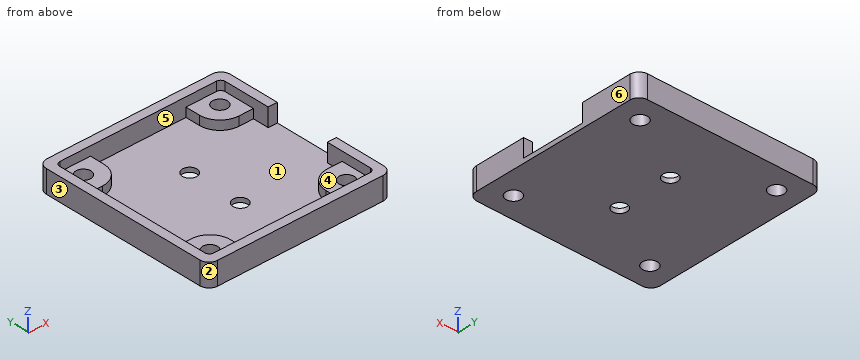
```python
from build123d import *

# Parameters (mm, degrees)
F0_R     = 1.6
F0_R_2   = 1.65
F0_W     = 2
F0_H     = 7
F1_DEPTH = 1
F2_DEPTH = 5
F3_DEPTH = 3
F4_R     = 2
F5_R     = 1


with BuildPart() as f1:
    # F0 (on Top) → F1 (new body)
    with BuildSketch(Plane.XY):
        with BuildLine():
            Line((-17.411994, -1.24302), (-17.411994, -4.438214))
            Line((-17.411994, -4.438214), (3.597618, -4.438214))
            Line((3.597618, -4.438214), (3.597618, -1.24302))
            ThreePointArc((3.597618, -1.24302), (4.915637, 1.93896), (8.097618, 3.25698))
            Line((8.097618, 3.25698), (11.292812, 3.25698))
            Line((11.292812, 3.25698), (11.292812, 6.761786))
            Line((11.292812, 6.761786), (11.292812, 13.761786))
            Line((11.292812, 13.761786), (11.292812, 20.761786))
            Line((11.292812, 20.761786), (11.292812, 24.266591))
            Line((11.292812, 24.266591), (8.097618, 24.266591))
            ThreePointArc((8.097618, 24.266591), (4.915637, 25.584611), (3.597618, 28.766591))
            Line((3.597618, 28.766591), (3.597618, 31.961786))
            Line((3.597618, 31.961786), (-17.411994, 31.961786))
            Line((-17.411994, 31.961786), (-17.411994, 28.766591))
            ThreePointArc((-17.411994, 28.766591), (-18.730013, 25.584611), (-21.911994, 24.266591))
            Line((-21.911994, 24.266591), (-25.107188, 24.266591))
            Line((-25.107188, 24.266591), (-25.107188, 3.25698))
            Line((-25.107188, 3.25698), (-21.911994, 3.25698))
            ThreePointArc((-21.911994, 3.25698), (-18.730013, 1.93896), (-17.411994, -1.24302))
        make_face()
        with Locations((-6.907188, 7.761786)):
            Circle(F0_R, mode=Mode.SUBTRACT)
        with Locations((-6.907188, 19.761786)):
            Circle(F0_R, mode=Mode.SUBTRACT)
        Polygon((-17.411994, -4.438214), (-25.107188, -4.438214), (-25.107188, 3.25698), (-25.107188, 24.266591), (-25.107188, 31.961786), (-17.411994, 31.961786), (3.597618, 31.961786), (11.292812, 31.961786), (11.292812, 24.266591), (11.292812, 20.761786), (13.292812, 20.761786), (13.292812, 33.961786), (-27.107188, 33.961786), (-27.107188, -6.438214), (13.292812, -6.438214), (13.292812, 6.761786), (11.292812, 6.761786), (11.292812, 3.25698), (11.292812, -4.438214), (3.597618, -4.438214), align=None)
        with BuildLine():
            Line((-25.107188, 31.961786), (-25.107188, 24.266591))
            Line((-25.107188, 24.266591), (-21.911994, 24.266591))
            ThreePointArc((-21.911994, 24.266591), (-18.730013, 25.584611), (-17.411994, 28.766591))
            Line((-17.411994, 28.766591), (-17.411994, 31.961786))
            Line((-17.411994, 31.961786), (-25.107188, 31.961786))
        make_face()
        with Locations((-21.911994, 28.766591)):
            Circle(F0_R_2, mode=Mode.SUBTRACT)
        with BuildLine():
            Line((11.292812, 31.961786), (3.597618, 31.961786))
            Line((3.597618, 31.961786), (3.597618, 28.766591))
            ThreePointArc((3.597618, 28.766591), (4.915637, 25.584611), (8.097618, 24.266591))
            Line((8.097618, 24.266591), (11.292812, 24.266591))
            Line((11.292812, 24.266591), (11.292812, 31.961786))
        make_face()
        with Locations((8.097618, 28.766591)):
            Circle(F0_R_2, mode=Mode.SUBTRACT)
        with Locations((12.292812, 17.261786)):
            Rectangle(F0_W, F0_H)
        with Locations((12.292812, 10.261786)):
            Rectangle(F0_W, F0_H)
    extrude(amount=F1_DEPTH)

    # F0 (on Top) → F2 (join)
    with BuildSketch(Plane.XY):
        Polygon((-17.411994, -4.438214), (-25.107188, -4.438214), (-25.107188, 3.25698), (-25.107188, 24.266591), (-25.107188, 31.961786), (-17.411994, 31.961786), (3.597618, 31.961786), (11.292812, 31.961786), (11.292812, 24.266591), (11.292812, 20.761786), (13.292812, 20.761786), (13.292812, 33.961786), (-27.107188, 33.961786), (-27.107188, -6.438214), (13.292812, -6.438214), (13.292812, 6.761786), (11.292812, 6.761786), (11.292812, 3.25698), (11.292812, -4.438214), (3.597618, -4.438214), align=None)
    extrude(amount=F2_DEPTH)

    # F0 (on Top) → F3 (join)
    with BuildSketch(Plane.XY):
        with BuildLine():
            Line((-25.107188, 31.961786), (-25.107188, 24.266591))
            Line((-25.107188, 24.266591), (-21.911994, 24.266591))
            ThreePointArc((-21.911994, 24.266591), (-18.730013, 25.584611), (-17.411994, 28.766591))
            Line((-17.411994, 28.766591), (-17.411994, 31.961786))
            Line((-17.411994, 31.961786), (-25.107188, 31.961786))
        make_face()
        with Locations((-21.911994, 28.766591)):
            Circle(F0_R_2, mode=Mode.SUBTRACT)
        with BuildLine():
            Line((-25.107188, 3.25698), (-25.107188, -4.438214))
            Line((-25.107188, -4.438214), (-17.411994, -4.438214))
            Line((-17.411994, -4.438214), (-17.411994, -1.24302))
            ThreePointArc((-17.411994, -1.24302), (-18.730013, 1.93896), (-21.911994, 3.25698))
            Line((-21.911994, 3.25698), (-25.107188, 3.25698))
        make_face()
        with Locations((-21.911994, -1.24302)):
            Circle(F0_R_2, mode=Mode.SUBTRACT)
        with BuildLine():
            Line((11.292812, 31.961786), (3.597618, 31.961786))
            Line((3.597618, 31.961786), (3.597618, 28.766591))
            ThreePointArc((3.597618, 28.766591), (4.915637, 25.584611), (8.097618, 24.266591))
            Line((8.097618, 24.266591), (11.292812, 24.266591))
            Line((11.292812, 24.266591), (11.292812, 31.961786))
        make_face()
        with Locations((8.097618, 28.766591)):
            Circle(F0_R_2, mode=Mode.SUBTRACT)
        with BuildLine():
            Line((3.597618, -1.24302), (3.597618, -4.438214))
            Line((3.597618, -4.438214), (11.292812, -4.438214))
            Line((11.292812, -4.438214), (11.292812, 3.25698))
            Line((11.292812, 3.25698), (8.097618, 3.25698))
            ThreePointArc((8.097618, 3.25698), (4.915637, 1.93896), (3.597618, -1.24302))
        make_face()
        with Locations((8.097618, -1.24302)):
            Circle(F0_R_2, mode=Mode.SUBTRACT)
    extrude(amount=F3_DEPTH)

    # F4
    f4_edges = [f1.edges().sort_by_distance(p)[0] for p in [
        (-27.107188, -6.438214, 2.5),
        (13.292812, -6.438214, 2.5),
        (13.292812, 33.961786, 2.5),
        (-27.107188, 33.961786, 2.5),
    ]]
    fillet(f4_edges, radius=F4_R)

    # F5
    f5_edges = [f1.edges().sort_by_distance(p)[0] for p in [
        (-25.107188, 31.961786, 4),
        (11.292812, 31.961786, 4),
        (11.292812, -4.438214, 4),
        (-25.107188, -4.438214, 4),
    ]]
    fillet(f5_edges, radius=F5_R)


solid = f1.part
```
Verification items for the finished model (mm, model axes). Face numbers are marked on the shaded views. A direction names the side the tool comes from. Coordinates: 2 decimals unless noted, no trailing zeros. Loops run counter-clockwise (first coordinate to the right, second up) from the corner with the lowest first, then second, coordinate; pieces in that order, holes last. Notation, with made-up numbers: (-25.5, 75) -> (-21.5, 75) arc R14 cw to (-21.5, 84) -> close; hole circle Ø11 at (62, 49.5). An arc over 180 degrees is marked (long way). Answer in a Markdown table with one row per item.
1) Draft check along Y on the marked faces 1, 2, 3 and 4. Enter one of: released by +Y, released by -Y, zero draft, split by the parting line, or undercut.
The answers:
| item | result |
|---|---|
| face 1 | undercut |
| face 2 | released by -Y |
| face 3 | zero draft |
| face 4 | undercut |
2) Access from +Z, -Z, +X, -X, +Y, -Y to the whole of each face (thin tool, end or side, straight path). Record for the marked faces 5 and 6.
The answers:
| item | result |
|---|---|
| face 5 | +Z |
| face 6 | +Z, -Z, +X, +Y, -Y |
3) Section check C-C (z = 4.1). Record the cut outline in (x, y), and give its area (3 significant figures).
The answers:
| item | result |
|---|---|
| outline | (-27.11, -4.44) arc R2 ccw to (-25.11, -6.44) -> (11.29, -6.44) arc R2 ccw to (13.29, -4.44) -> (13.29, 6.76) -> (11.29, 6.76) -> (11.29, -3.44) arc R1 cw to (10.29, -4.44) -> (-24.11, -4.44) arc R1 cw to (-25.11, -3.44) -> (-25.11, 30.96) arc R1 cw to (-24.11, 31.96) -> (10.29, 31.96) arc R1 cw to (11.29, 30.96) -> (11.29, 20.76) -> (13.29, 20.76) -> (13.29, 31.96) arc R2 ccw to (11.29, 33.96) -> (-25.11, 33.96) arc R2 ccw to (-27.11, 31.96) -> close |
| area | 277 mm2 |
4) Scan lines: line 1 along Y through (x, z) = (10, 2.5); line 2 along X through (y, z) = (29, 3.9); line 3 along Y through (x, z) = (-17, 2.7). Record each from-to range of solid material in increasing order. Write a range as from..to.
The answers:
| item | result |
|---|---|
| line 1 | y = -6.44..3.26, 24.27..33.96 |
| line 2 | x = -27.11..-25.11, 11.29..13.29 |
| line 3 | y = -6.44..-4.44, 31.96..33.96 |
5) Section check B-B (x = -10). Record the cut outline in (y, z).
The answers:
| item | result |
|---|---|
| outline | (-6.44, 0) -> (33.96, 0) -> (33.96, 5) -> (31.96, 5) -> (31.96, 1) -> (-4.44, 1) -> (-4.44, 5) -> (-6.44, 5) -> close |
6) Section check A-A (z = 1.9). Give the number of separate pieces and of enclosed holes in the cut face, and give its area (3 significant figures).
The answers:
| item | result |
|---|---|
| separate pieces | 1 |
| enclosed holes | 4 |
| area | 461 mm2 |
7) Depth check by flat-ended pin: P1, Ø1, axis at y = 10.5, z = 3, coming from the +X side; P2, Ø3, axis at x = -21.91, y = -1.24, coming from the +Z side. Enter the tip coordinate at first touch or a pass-through.
The answers:
| item | result |
|---|---|
| P1 | stops at x = -25.11 |
| P2 | passes through |
8) Section check D-D (y = 23). Record the cut outline in (x, z), and give its area (3 significant figures).
The answers:
| item | result |
|---|---|
| outline | (-27.11, 0) -> (13.29, 0) -> (13.29, 5) -> (11.29, 5) -> (11.29, 1) -> (-25.11, 1) -> (-25.11, 5) -> (-27.11, 5) -> close |
| area | 56.4 mm2 |
